Source: CAD feature listing. Evaluate the final solid. Frame: model axes, mm. A direction names the side the tool comes from. Round coordinates to 2 decimals unless told otherwise and drop trailing zeros. Write each loop counter-clockwise with the first axis right and the second up, starting at its lowest first coordinate (ties: lowest second). Pieces come first, ordered by that corner, then holes.
from build123d import *

# Parameters (mm, degrees)
SKETCH1_R           = 25.4
BOSS_EXTRUDE1_DEPTH = 3.175
SKETCH2_R           = 22.225
BOSS_EXTRUDE2_DEPTH = 12.7
SKETCH3_R           = 9.525
CUT_EXTRUDE1_DEPTH  = 16.875
CHAMFER1_SIZE       = 1
CHAMFER1_SIZE2      = 0.176326981
CHAMFER2_SIZE       = 1.5


with BuildPart() as part:
    # Sketch1 → Boss-Extrude1 (new body)
    with BuildSketch(Plane(origin=(0, 0, 0), x_dir=(0, 0, -1), z_dir=(1, 0, 0))):
        Circle(SKETCH1_R)
    extrude(amount=BOSS_EXTRUDE1_DEPTH)

    # Sketch2 → Boss-Extrude2 (add)
    with BuildSketch(Plane(origin=(3.175, 0, 0), x_dir=(0, 0, -1), z_dir=(1, 0, 0))):
        Circle(SKETCH2_R)
    extrude(amount=BOSS_EXTRUDE2_DEPTH)

    # Sketch3 → Cut-Extrude1 (cut, through all)
    with BuildSketch(Plane.ZY):
        Circle(SKETCH3_R)
    extrude(amount=-CUT_EXTRUDE1_DEPTH, mode=Mode.SUBTRACT)

    # Chamfer1
    chamfer1_edges = [part.edges().sort_by_distance(p)[0] for p in [
        (15.875, 0, 22.225),
    ]]
    chamfer1_side = [part.faces().sort_by_distance(p)[0] for p in [
        (9.525, 0, 22.225),
    ]]
    chamfer(chamfer1_edges, length=CHAMFER1_SIZE, length2=CHAMFER1_SIZE2, reference=chamfer1_side[0])

    # Chamfer2
    chamfer2_edges = [part.edges().sort_by_distance(p)[0] for p in [
        (3.175, 0, 25.4),
    ]]
    chamfer(chamfer2_edges, length=CHAMFER2_SIZE)


solid = part.part
1) Contact query for flat-ended pins moving along their axis: P1, Ø3, axis at x = 13, z = -6.5, coming from the -Y side; P2, Ø17, axis at y = 0, z = 0, coming from the +X side (3 decimals); P3, Ø5, axis at x = 6, z = 18.5, coming from the +Y side; P4, Ø1, axis at x = 7.5, z = 11, coming from the +Y side. Output: stop coordinate, or through.
Taken from the geometry:
P1: stops at y = -21.66
P2: passes through
P3: stops at y = 15.43
P4: stops at y = 19.59
2) Material intervals for line 1 (Y direction, x = 6, z = 0) (3 decimals); line 2 (Y direction, x = 5.75, z = -7); line 3 (X direction, y = 13.5, z = -18.5) (3 decimals), sorted ascending.
Taken from the geometry:
line 1: y = -22.225 to -9.525, 9.525 to 22.225
line 2: y = -21.09 to -6.46, 6.46 to 21.09
line 3: x = 0 to 3.175
3) Reachability of faces 1 (the face through (8.943, 6.676, -21.199)), 2 (the face through (0, 0, -11)) from +Z, -Z, +X, -X, +Y, -Y: full face, straight path, thin tool, end or side. Return the list, or none.
Taken from the geometry:
face 1: +X
face 2: +Z, -Z, -X, +Y, -Y
4) Pull-direction query (Z, two-part tool) for faces 3 (the face through (0.826, -24.796, 5.506)), 4 (the face through (15.875, -5, -9)), 5 (the face through (7.826, -5.796, -7.559)); classes: released by +Z, released by -Z, zero draft, split by the parting line, or undercut.
Taken from the geometry:
face 3: split by the parting line
face 4: zero draft
face 5: undercut
5) Section query C-C on x = 6.5. Return the cut outline in (y, z) (3 decimals).
Taken from the geometry:
outline: circle Ø44.45 at (0, 0); hole circle Ø19.05 at (0, 0)
6) Section query A-A on y = 0. Return the cut outline in (x, z) (3 decimals), then the cut area to 3 significant figures.
Taken from the geometry:
outline: (0, -25.4) - (1.675, -25.4) - (3.175, -23.9) - (3.175, -22.225) - (14.875, -22.225) - (15.875, -22.049) - (15.875, -9.525) - (0, -9.525) - close; (0, 9.525) - (15.875, 9.525) - (15.875, 22.049) - (14.875, 22.225) - (3.175, 22.225) - (3.175, 23.9) - (1.675, 25.4) - (0, 25.4) - close
area: 421 mm2
